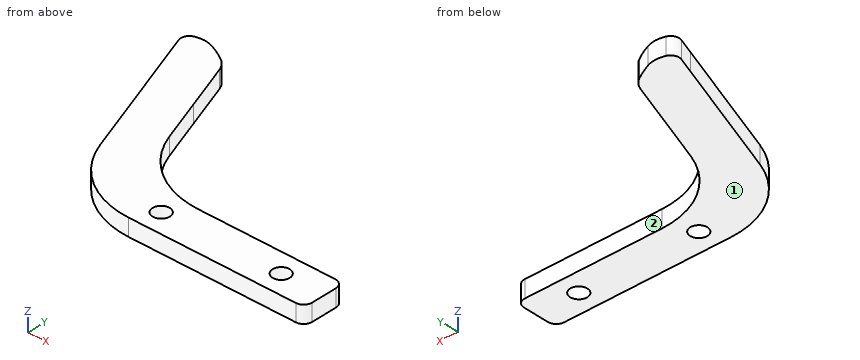
```python
from build123d import *

# Parameters (mm, degrees)
SKETCH_1_W      = 50
SKETCH_1_H      = 10
SKETCH_1_R      = 2
SKETCH_1_W_2    = 5
EXTRUDE_1_DEPTH = 4
FILLET_1_R      = 20
FILLET_2_R      = 20
FILLET_3_R      = 2
EXTRUDE_2_DEPTH = 4


with BuildPart() as part:
    # 草图1 → 凸台-拉伸1 (new body)
    with BuildSketch(Plane.XY):
        Polygon((-49.968629634, 37.889241728), (-61.844641091, 41.280271037), (-45, -5), (-45, 5), (-37.997924618, 5), align=None)
        with Locations((-20, 0)):
            Rectangle(SKETCH_1_W, SKETCH_1_H)
        with Locations((-28, 0)):
            Circle(SKETCH_1_R, mode=Mode.SUBTRACT)
        Circle(SKETCH_1_R, mode=Mode.SUBTRACT)
        with Locations((7.5, 0)):
            Rectangle(SKETCH_1_W_2, SKETCH_1_H)
    extrude(amount=EXTRUDE_1_DEPTH)

    # 圆角1
    fillet_1_edges = [part.edges().sort_by_distance(p)[0] for p in [
        (-37.997924618, 5, 2),
        (-45, -5, 2),
    ]]
    fillet(fillet_1_edges, radius=FILLET_1_R)

    # 圆角2
    fillet_2_edges = [part.edges().sort_by_distance(p)[0] for p in [
        (-49.968629634, 37.889241728, 2),
    ]]
    fillet(fillet_2_edges, radius=FILLET_2_R)

    # 圆角3
    fillet_3_edges = [part.edges().sort_by_distance(p)[0] for p in [
        (-61.844641091, 41.280271037, 2),
        (10, -5, 2),
        (10, 5, 2),
    ]]
    fillet(fillet_3_edges, radius=FILLET_3_R)

    # 草图2 → 凸台-拉伸2 (add)
    with BuildSketch(Plane.XY.offset(4)):
        with BuildLine():
            ThreePointArc((-56.355465994, 43.741712807), (-58.489892138, 44.170450367), (-60.636797067, 43.809354689))
            ThreePointArc((-60.636797067, 43.809354689), (-61.765372114, 42.775205935), (-61.832141712, 41.245929274))
            Line((-61.832141712, 41.245929274), (-60.464061138, 37.487158791))
            ThreePointArc((-60.464061138, 37.487158791), (-60.461686369, 38.861729082), (-59.572682652, 39.910119045))
            ThreePointArc((-59.572682652, 39.910119045), (-59.555544901, 39.941826673), (-59.538179031, 39.973409941))
            ThreePointArc((-59.538179031, 39.973409941), (-59.402093878, 40.007270752), (-59.26871602, 40.050584379))
            ThreePointArc((-59.26871602, 40.050584379), (-58.553081169, 40.170949505), (-57.841605929, 40.028036987))
            ThreePointArc((-57.841605929, 40.028036987), (-50.908526864, 35.37662093), (-46.47845319, 28.300060756))
            Line((-46.47845319, 28.300060756), (-50.467059195, 39.258665691))
            ThreePointArc((-50.467059195, 39.258665691), (-51.276051122, 40.690541098), (-52.50584262, 41.782487979))
            ThreePointArc((-52.50584262, 41.782487979), (-54.386487154, 42.848883136), (-56.355465994, 43.741712807))
        make_face()
    extrude(amount=-EXTRUDE_2_DEPTH)


solid = part.part
```
Verification items for the finished model (mm, model axes). Face numbers are marked on the shaded views. A direction names the side the tool comes from. Coordinates: 2 decimals unless noted, no trailing zeros. Loops run counter-clockwise (first coordinate to the right, second up) from the corner with the lowest first, then second, coordinate; pieces in that order, holes last. Notation, with made-up numbers: (53, -20.75) -> (110, -20.75) arc R22 cw to (110, -1.75) -> close; hole circle Ø3 at (37, 22.25). An arc over 180 degrees is marked (long way). Answer in a Markdown table with one row per item. Add a question column.
1. Section check A-A, the plane x = 0. Enter the section's corners in (y, z).
2. Depth check by flat-ended pin: P1, Ø6.5, axis at x = 0, y = 0, coming from the -Z side; P2, Ø1.2, axis at x = -10, z = 1.5, coming from the +Y side; P3, Ø1.5, axis at y = 36.5, z = 2.5, coming from the +X side. Enter the tip coordinate at first touch or a pass-through.
3. Section check B-B, the plane y = 0. Enter the section's corners in (x, z), then the cut area to 3 significant figures.
4. Section check D-D, the plane z = 2.15. Give the number of separate pieces and of enclosed holes in the cut face, then the cut area to 3 significant figures.
5. Access from +Z, -Z, +X, -X, +Y, -Y to the whole of each face (thin tool, end or side, straight path). Record for the marked faces 1 and 2.
6. Material ranges on probe 1 along Y at (x, z) = (0, 3.05); probe 2 along Y at (x, z) = (-8.5, 3.25); probe 3 along Y at (x, z) = (-28, 3), recorded low to high. Write a range as [from, to].
7. Section check C-C, the plane x = -18.5. Enter the section's corners in (y, z), then the cut area to 3 significant figures.
Derived:
| question | item | result |
|---|---|---|
| 1 | outline | (-5, 0) -> (-2, 0) -> (-2, 4) -> (-5, 4) -> close; (2, 0) -> (5, 0) -> (5, 4) -> (2, 4) -> close |
| 2 | P1 | stops at z = 0 |
| 2 | P2 | stops at y = 5 |
| 2 | P3 | stops at x = -49.19 |
| 3 | outline | (-44.22, 0) -> (-30, 0) -> (-30, 4) -> (-44.22, 4) -> close; (-26, 0) -> (-2, 0) -> (-2, 4) -> (-26, 4) -> close; (2, 0) -> (10, 0) -> (10, 4) -> (2, 4) -> close |
| 3 | area | 185 mm² |
| 4 | separate pieces | 1 |
| 4 | enclosed holes | 3 |
| 4 | area | 948 mm² |
| 5 | face 1 | -Z, +X, -X, +Y, -Y |
| 5 | face 2 | +Z, -Z, +X, +Y |
| 6 | probe 1 | y = [-5, -2], [2, 5] |
| 6 | probe 2 | y = [-5, 5] |
| 6 | probe 3 | y = [-5, -2], [2, 5.41] |
| 7 | outline | (-5, 0) -> (5, 0) -> (5, 4) -> (-5, 4) -> close |
| 7 | area | 40.0 mm² |
